```python
from build123d import *

# Parameters (mm, degrees)
ESQUISSE1_W        = 155
ESQUISSE1_H        = 61
ESQUISSE1_R        = 5
ESQUISSE1_R_2      = 1.5
BOSS_EXTRU_2_DEPTH = 2


with BuildPart() as part:
    # Esquisse1 → Boss.-Extru.2 (new body)
    with BuildSketch(Plane(origin=(0, 0, 0), x_dir=(1, 0, 0), z_dir=(0, 1, 0))):
        Rectangle(ESQUISSE1_W, ESQUISSE1_H)
        with Locations((-52.5, 14.5)):
            Circle(ESQUISSE1_R, mode=Mode.SUBTRACT)
        with Locations((-37.5, 14.5)):
            Circle(ESQUISSE1_R, mode=Mode.SUBTRACT)
        with Locations((-22.5, 14.5)):
            Circle(ESQUISSE1_R, mode=Mode.SUBTRACT)
        with Locations((-7.5, 14.5)):
            Circle(ESQUISSE1_R, mode=Mode.SUBTRACT)
        with Locations((7.5, 14.5)):
            Circle(ESQUISSE1_R, mode=Mode.SUBTRACT)
        with Locations((22.5, 14.5)):
            Circle(ESQUISSE1_R, mode=Mode.SUBTRACT)
        with Locations((37.5, 14.5)):
            Circle(ESQUISSE1_R, mode=Mode.SUBTRACT)
        with Locations((52.5, 14.5)):
            Circle(ESQUISSE1_R, mode=Mode.SUBTRACT)
        with Locations((-37.5, -0.5)):
            Circle(ESQUISSE1_R, mode=Mode.SUBTRACT)
        with Locations((-22.5, -0.5)):
            Circle(ESQUISSE1_R, mode=Mode.SUBTRACT)
        with Locations((-7.5, -0.5)):
            Circle(ESQUISSE1_R, mode=Mode.SUBTRACT)
        with Locations((7.5, -0.5)):
            Circle(ESQUISSE1_R, mode=Mode.SUBTRACT)
        with Locations((22.5, -0.5)):
            Circle(ESQUISSE1_R, mode=Mode.SUBTRACT)
        with Locations((37.5, -0.5)):
            Circle(ESQUISSE1_R, mode=Mode.SUBTRACT)
        with Locations((52.5, -0.5)):
            Circle(ESQUISSE1_R, mode=Mode.SUBTRACT)
        with Locations((-52.5, -0.5)):
            Circle(ESQUISSE1_R, mode=Mode.SUBTRACT)
        with Locations((-52.5, 25.5)):
            Circle(ESQUISSE1_R_2, mode=Mode.SUBTRACT)
        with Locations((-37.5, 25.5)):
            Circle(ESQUISSE1_R_2, mode=Mode.SUBTRACT)
        with Locations((-22.5, 25.5)):
            Circle(ESQUISSE1_R_2, mode=Mode.SUBTRACT)
        with Locations((-7.5, 25.5)):
            Circle(ESQUISSE1_R_2, mode=Mode.SUBTRACT)
        with Locations((7.5, 25.5)):
            Circle(ESQUISSE1_R_2, mode=Mode.SUBTRACT)
        with Locations((22.5, 25.5)):
            Circle(ESQUISSE1_R_2, mode=Mode.SUBTRACT)
        with Locations((37.5, 25.5)):
            Circle(ESQUISSE1_R_2, mode=Mode.SUBTRACT)
        with Locations((52.5, 25.5)):
            Circle(ESQUISSE1_R_2, mode=Mode.SUBTRACT)
        with Locations((-52.5, -11.5)):
            Circle(ESQUISSE1_R_2, mode=Mode.SUBTRACT)
        with Locations((-37.5, -11.5)):
            Circle(ESQUISSE1_R_2, mode=Mode.SUBTRACT)
        with Locations((-22.5, -11.5)):
            Circle(ESQUISSE1_R_2, mode=Mode.SUBTRACT)
        with Locations((-7.5, -11.5)):
            Circle(ESQUISSE1_R_2, mode=Mode.SUBTRACT)
        with Locations((7.5, -11.5)):
            Circle(ESQUISSE1_R_2, mode=Mode.SUBTRACT)
        with Locations((22.5, -11.5)):
            Circle(ESQUISSE1_R_2, mode=Mode.SUBTRACT)
        with Locations((37.5, -11.5)):
            Circle(ESQUISSE1_R_2, mode=Mode.SUBTRACT)
        with Locations((52.5, -11.5)):
            Circle(ESQUISSE1_R_2, mode=Mode.SUBTRACT)
        with Locations((46.5, -27)):
            Circle(ESQUISSE1_R_2, mode=Mode.SUBTRACT)
        with Locations((-72.5, 25.5)):
            Circle(ESQUISSE1_R_2, mode=Mode.SUBTRACT)
        with Locations((-72.5, -25.5)):
            Circle(ESQUISSE1_R_2, mode=Mode.SUBTRACT)
        with Locations((72.5, 25.5)):
            Circle(ESQUISSE1_R_2, mode=Mode.SUBTRACT)
    extrude(amount=BOSS_EXTRU_2_DEPTH)


solid = part.part
```
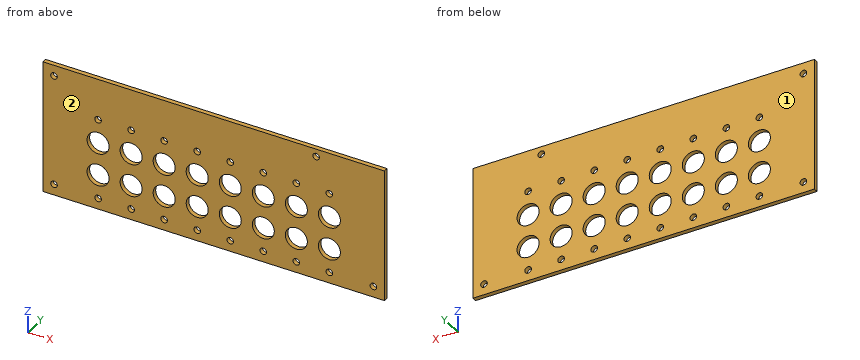
Geometry check sheet. Reference: the model listing, model coordinates, mm. Face numbers are marked on the shaded views. Coordinates: 2 decimals unless noted, no trailing zeros. Write each loop counter-clockwise with the first axis right and the second up, starting at its lowest first coordinate (ties: lowest second). Pieces come first, ordered by that corner, then holes. Notation, with made-up numbers: M 70,-37.5 L 92,-37.5 A27 ccw 92,-11.5 Z; hole C 13.5,-11.75 d2. An arc over 180 degrees is marked long. Use one line per item in the form item = value. Start each with the question number.
1) Release check for a two-part mould opening along Y. For the marked faces 1 and 2 record: pulls with the +Y half, pulls with the -Y half, needs draft (parallel to the pull), parting line crosses it, or undercut.
2) Section check D-D on y = 0.9. State how many separate pieces and enclosed holes the cut face has, and give its area (3 significant figures).
3) Section check B-B on x = 72.5. Enter the section's corners in (y, z), and give its area (3 significant figures).
4) Section check A-A on x = -72.5. Enter the section's corners in (y, z), and give its area (3 significant figures).
5) Section check C-C on x = 22.5. Enter the section's corners in (y, z).
6) Thickness scan on probe 1 along Z at (x, y) = (52.5, 1); probe 2 along Z at (x, y) = (9.5, 0.6); probe 3 along Z at (x, y) = (40.5, 1.5). Record the ranges inside material, lowest first. Write a range as from..to.
Responses:
q1.face_1 = pulls with the +Y half
q1.face_2 = pulls with the -Y half
q2.separate_pieces = 1
q2.enclosed_holes = 36
q2.area = 8,060 mm2
q3.outline = M 0,-30.5 L 2,-30.5 L 2,-27 L 0,-27 Z; M 0,-24 L 2,-24 L 2,30.5 L 0,30.5 Z
q3.area = 116 mm2
q4.outline = M 0,-30.5 L 2,-30.5 L 2,-27 L 0,-27 Z; M 0,-24 L 2,-24 L 2,24 L 0,24 Z; M 0,27 L 2,27 L 2,30.5 L 0,30.5 Z
q4.area = 110 mm2
q5.outline = M 0,-30.5 L 2,-30.5 L 2,-27 L 0,-27 Z; M 0,-24 L 2,-24 L 2,-19.5 L 0,-19.5 Z; M 0,-9.5 L 2,-9.5 L 2,-4.5 L 0,-4.5 Z; M 0,5.5 L 2,5.5 L 2,10 L 0,10 Z; M 0,13 L 2,13 L 2,30.5 L 0,30.5 Z
q6.probe_1 = -30.5..-27, -24..-19.5, -9.5..-4.5, 5.5..10, 13..30.5
q6.probe_2 = -30.5..-19.08, -9.92..-4.08, 5.08..30.5
q6.probe_3 = -30.5..-18.5, -10.5..-3.5, 4.5..30.5
